Can you work these out from the model? Positions are in its coordinate system, mm. A direction names the side the tool comes from. Round coordinates to 2 decimals unless told otherwise and drop trailing zeros. Loops run counter-clockwise (first coordinate to the right, second up) from the corner with the lowest first, then second, coordinate; pieces in that order, holes last. Notation, with made-up numbers: M -4.5,-6 L 44.5,-6 A27 ccw 44.5,26 Z; hole C 50,64 d3. An arc over 180 degrees is marked long. Return JSON: item names as keys, results as strings.
```python
from build123d import *

# Parameters (mm, degrees)
SKETCH_2_W = 40
SKETCH_2_H = 2.5
FILLET_1_R = 2.5
FILLET_2_R = 2.5
FILLET_3_R = 2.5


with BuildPart() as part:
    # 扫描1: sweep along a path in 草图3
    with BuildLine(Plane.XY) as sweep_1_path:
        Line((21.74, 20), (21.74, 0))
        Line((21.74, 0), (0, 0))
        Line((0, 0), (-21.74, 0))
        Line((-21.74, 0), (-21.74, -20))
    # 草图2 → 扫描1 (sweep)
    with BuildSketch(Plane(origin=(0, 0, 0), x_dir=(0, 0, -1), z_dir=(1, 0, 0))):
        Rectangle(SKETCH_2_W, SKETCH_2_H)
    sweep(path=sweep_1_path.line, transition=Transition.RIGHT)

    # 圆角1
    fillet_1_edges = [part.edges().sort_by_distance(p)[0] for p in [
        (-22.99, 1.25, 0),
    ]]
    fillet(fillet_1_edges, radius=FILLET_1_R)

    # 圆角2
    fillet_2_edges = [part.edges().sort_by_distance(p)[0] for p in [
        (22.99, -1.25, 0),
    ]]
    fillet(fillet_2_edges, radius=FILLET_2_R)

    # 圆角3
    fillet_3_edges = [part.edges().sort_by_distance(p)[0] for p in [
        (-20.49, -1.25, 0),
        (20.49, 1.25, 0),
    ]]
    fillet(fillet_3_edges, radius=FILLET_3_R)


solid = part.part
```
Q1. Suppose I cut it at B-B, the plane x = -8. Please give me the cut outline in (y, z).
Results:
{"outline": "M -1.25,-20 L 1.25,-20 L 1.25,20 L -1.25,20 Z"}
Q2. I'm going to push flat-ended pins straight in: pin 1 Ø8 at (y, z) = (-11, -5.5) entering from +X; pin 2 Ø11.5 at (x, z) = (0.5, 7.5) entering from +Y; pin 3 Ø19 at (x, z) = (-1, 0.5) entering from -Y. Where does each tip first touch, or does it pass through?
Results:
{"pin 1": "stops at x = -20.49", "pin 2": "stops at y = 1.25", "pin 3": "stops at y = -1.25"}
Q3. Suppose I cut it at A-A, the plane z = -10. Please give me the cut outline in (x, y).
Results:
{"outline": "M -22.99,-20 L -20.49,-20 L -20.49,-3.75 A2.5 cw -17.99,-1.25 L 20.49,-1.25 A2.5 ccw 22.99,1.25 L 22.99,20 L 20.49,20 L 20.49,3.75 A2.5 cw 17.99,1.25 L -20.49,1.25 A2.5 ccw -22.99,-1.25 Z"}
Q4. If I drill on line 1 along X through (y, z) = (4.5, -5.5); line 2 along Y through (x, z) = (-7, 5); line 3 along X through (y, z) = (-10.5, 4), over which ranges is the centre line in solid material (lowest first)?
Results:
{"line 1": "x = 20.49 to 22.99", "line 2": "y = -1.25 to 1.25", "line 3": "x = -22.99 to -20.49"}
Q5. On a 3-axis mill with a long thin cutter (end or side, diameter ignored), from which of +Z, -Z, +X, -X, +Y, -Y can I reach the whole of each face in a straight line? I mean faces 1 (the flat face through (-22, -20, 0)), 2 (the flat face through (-2, 1.25, 0)), 3 (the flat face through (1, -1.25, 0)). Say none if no direction works.
Results:
{"face 1": "+Z, -Z, +X, -X, -Y", "face 2": "+Z, -Z, -X, +Y", "face 3": "+Z, -Z, +X, -Y"}
Q6. Suppose I cut it at C-C, the plane y = 13. Please give me the cut outline in (x, z), plus the area to 3 significant figures.
Results:
{"outline": "M 20.49,-20 L 22.99,-20 L 22.99,20 L 20.49,20 Z", "area": "100 mm2"}
